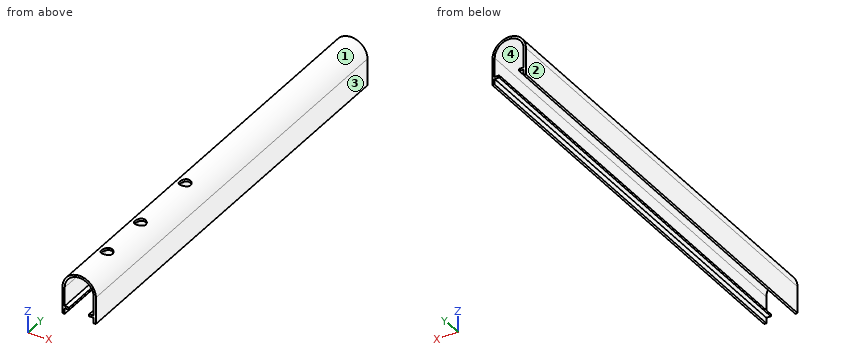
```python
from build123d import *

# Parameters (mm, degrees)
BOSS_EXTRU_1_DEPTH      = 200
ENL_V_MAT_EXTRU_1_DEPTH = 202.088289067
ESQUISSE6_R             = 2.5
ENL_V_MAT_EXTRU_3_DEPTH = 202.088289067


with BuildPart() as part:
    # Esquisse1 → Boss.-Extru.1 (new body)
    with BuildSketch(Plane(origin=(0, 0, 0), x_dir=(1, 0, 0), z_dir=(0, 1, 0))):
        with BuildLine():
            Line((-7.5, 0), (7.5, 0))
            Line((7.5, 0), (7.5, -12))
            ThreePointArc((7.5, -12), (0, -19.5), (-7.5, -12))
            Line((-7.5, -12), (-7.5, 0))
        make_face()
    extrude(amount=BOSS_EXTRU_1_DEPTH)

    # Esquisse2 → Enlèv. mat.-Extru.1 (cut, through all)
    with BuildSketch(Plane(origin=(0, 200, 0), x_dir=(1, 0, 0), z_dir=(0, 1, 0))):
        with BuildLine():
            Line((-6.5, 2.5), (6.5, 2.5))
            Line((6.5, 2.5), (6.5, -2.5))
            Line((6.5, -2.5), (4.5, -2.5))
            Line((4.5, -2.5), (4.5, -3.5))
            Line((4.5, -3.5), (6.5, -3.5))
            Line((6.5, -3.5), (6.5, -12))
            ThreePointArc((6.5, -12), (0, -18.5), (-6.5, -12))
            Line((-6.5, -12), (-6.5, -3.5))
            Line((-6.5, -3.5), (-4.5, -3.5))
            Line((-4.5, -3.5), (-4.5, -2.5))
            Line((-4.5, -2.5), (-6.5, -2.5))
            Line((-6.5, -2.5), (-6.5, 2.5))
        make_face()
    extrude(amount=-ENL_V_MAT_EXTRU_1_DEPTH, mode=Mode.SUBTRACT)

    # Esquisse6 → Enlèv. mat.-Extru.3 (cut, through all)
    with BuildSketch(Plane.XY):
        with Locations(Location((0, 20.5, 0), (0, 0, 180))):
            Circle(ESQUISSE6_R)
        with Locations(Location((0, 45, 0), (0, 0, 180))):
            Circle(ESQUISSE6_R)
        with Locations(Location((0, 78, 0), (0, 0, 180))):
            Circle(ESQUISSE6_R)
    extrude(amount=ENL_V_MAT_EXTRU_3_DEPTH, mode=Mode.SUBTRACT)


solid = part.part
```
Input: part model. Units: mm. Frame: model coordinates. Face numbers are marked on the shaded views. Give positions to 0.01 mm unless a question says otherwise; leave off trailing zeros. Order: outer loops, then holes, each group sorted by start corner. A loop starts at its lowest first (then second) coordinate and runs counter-clockwise, first axis right, second up. Notation, with made-up numbers: (-2.5, 13) - (37.5, 13) arc R24 cw to (37.5, 23) - close; hole circle Ø3 at (42, 48.5). An arc over 180 degrees is marked (long way). Put each result on its own line as item: value.
Item 1: Section query B-B, the plane y = 175.5. Return loops of the section in (x, z).
Found:
outline: (-7.5, 0) - (-6.5, 0) - (-6.5, 2.5) - (-4.5, 2.5) - (-4.5, 3.5) - (-6.5, 3.5) - (-6.5, 12) arc R6.5 cw to (6.5, 12) - (6.5, 3.5) - (4.5, 3.5) - (4.5, 2.5) - (6.5, 2.5) - (6.5, 0) - (7.5, 0) - (7.5, 12) arc R7.5 ccw to (-7.5, 12) - close
Item 2: Contact query for flat-ended pins moving along their axis: pin 1 (1.6 mm diameter, centred on x = 5.5, y = 98.5, fed in from +Z); pin 2 (6.5 mm diameter, centred on x = 0, y = 20.5, fed in from -Z); pin 3 (1 mm diameter, centred on x = 5, y = 106, fed in from -Z). Output: stop coordinate, or through.
Found:
pin 1: stops at z = 17.84
pin 2: stops at z = 17.63
pin 3: stops at z = 2.5
Item 3: Ray query, L1, parallel to X at y = 108.5, z = 8.5; L2, parallel to X at y = 126, z = 2.75; L3, parallel to Z at x = 4.75, y = 116.5. Return the intervals inside material, ascending. Write a range as from..to.
Found:
L1: x = -7.5..-6.5, 6.5..7.5
L2: x = -7.5..-4.5, 4.5..7.5
L3: z = 2.5..3.5, 16.44..17.8
Item 4: Section query C-C, the plane z = 15. Return loops of the section in (x, y), then the cut area to 3 significant figures.
Found:
outline: (-6.87, 0) - (-5.77, 0) - (-5.77, 200) - (-6.87, 200) - close; (5.77, 0) - (6.87, 0) - (6.87, 200) - (5.77, 200) - close
area: 443 mm^2
Item 5: Draft query along X for the marked faces 1, 2, 3 and 4. Return one class per face: +X half, -X half, draft (parallel to the pull), parting line (faces both ways), or undercut.
Found:
face 1: parting line
face 2: -X half
face 3: +X half
face 4: undercut
Item 6: Section query A-A, the plane y = 45. Return loops of the section in (x, z).
Found:
outline: (-7.5, 0) - (-6.5, 0) - (-6.5, 2.5) - (-4.5, 2.5) - (-4.5, 3.5) - (-6.5, 3.5) - (-6.5, 12) arc R6.5 cw to (-2.5, 18) - (-2.5, 19.07) arc R7.5 ccw to (-7.5, 12) - close; (2.5, 18) arc R6.5 cw to (6.5, 12) - (6.5, 3.5) - (4.5, 3.5) - (4.5, 2.5) - (6.5, 2.5) - (6.5, 0) - (7.5, 0) - (7.5, 12) arc R7.5 ccw to (2.5, 19.07) - close
